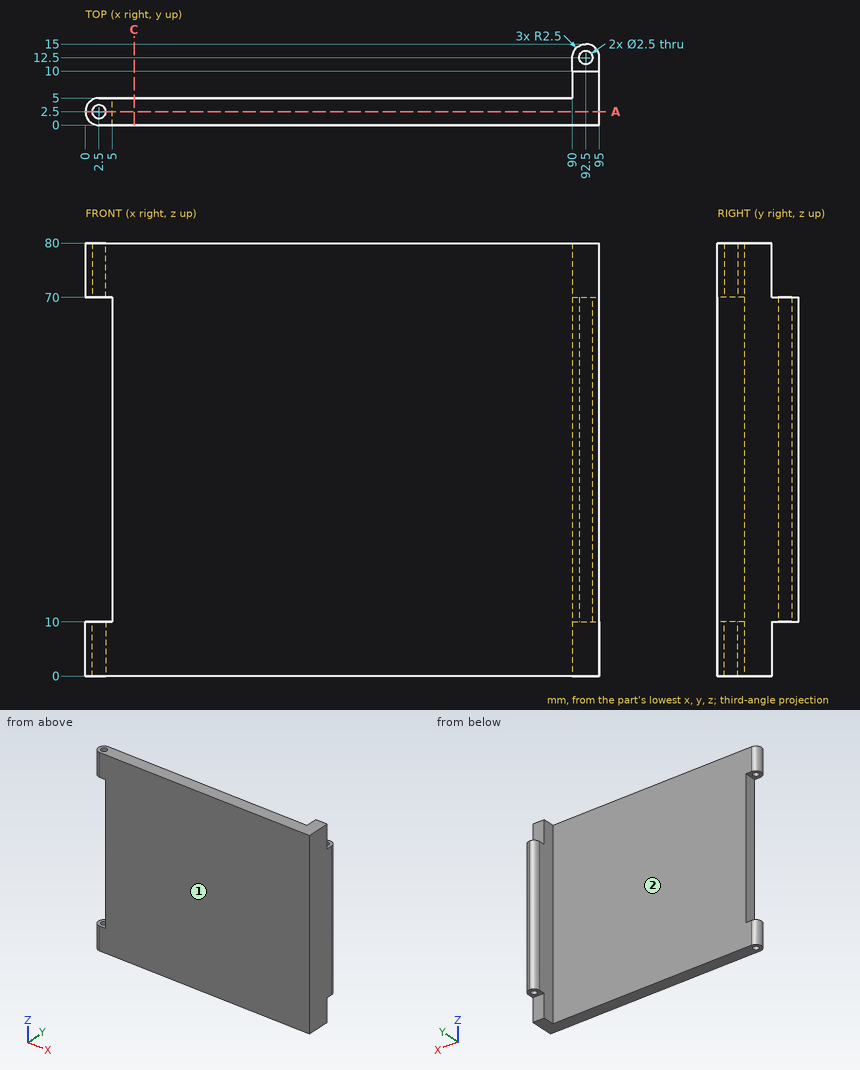
Can you work these out from the drawing? Everything is in mm from the part's minimum corner. A direction names the side the tool comes from. Round coordinates to 2 decimals unless told otherwise and drop trailing zeros. Loops run counter-clockwise (first coordinate to the right, second up) from the corner with the lowest first, then second, coordinate; pieces in that order, holes last. Notation, with made-up numbers: (46, 21.25) -> (95, 21.25) arc R19 ccw to (95, 49.25) -> close; hole circle Ø11 at (36, -4.75). An arc over 180 degrees is marked (long way). Use CSV: the item, a comma, the result in double quotes.
(1) If I drill on probe 1 along X at (y, z) = (9.25, 27.5); probe 2 along X at (y, z) = (12.5, 47); probe 3 along Y at (x, z) = (92.5, 48.5), over which ranges is the centre line in solid material (lowest first)? Write a range as [from, to].
Return value:
probe 1,"x = [90, 95]"
probe 2,"x = [90, 91.25], [93.75, 95]"
probe 3,"y = [0, 11.25], [13.75, 15]"
(2) For the marked faces 1 and 2, which set-ups out of +Z, -Z, +X, -X, +Y, -Y let a thin tool reach every point of the face, with its end or its side?
Return value:
face 1,"+Z, -Z, +X, -X, -Y"
face 2,"+Z, -Z, -X, +Y"
(3) Suppose I cut it at C-C on x = 9. Write out the boundary of the cut face in (y, z).
Return value:
outline,"(0, 0) -> (5, 0) -> (5, 80) -> (0, 80) -> close"
(4) Will these pins go through, and if not, where does the flat tip stop? pin 1 Ø5 at (y, z) = (12, 30.5) entering from -X; pin 2 Ø5.5 at (y, z) = (2, 37) entering from -X; pin 3 Ø6 at (x, z) = (27, 58.5) entering from +Y.
Return value:
pin 1,"stops at x = 90"
pin 2,"stops at x = 5"
pin 3,"stops at y = 5"
(5) Suppose I cut it at A-A on y = 2.5. Write out the boundary of the cut face in (x, z).
Return value:
outline,"(0, 0) -> (1.25, 0) -> (1.25, 10) -> (0, 10) -> close; (0, 70) -> (1.25, 70) -> (1.25, 80) -> (0, 80) -> close; (3.75, 0) -> (95, 0) -> (95, 80) -> (3.75, 80) -> (3.75, 70) -> (5, 70) -> (5, 10) -> (3.75, 10) -> close"
